Input: part model. Units: mm. Frame: model coordinates. Face numbers are marked on the shaded views. A direction names the side the tool comes from. Round coordinates to 2 decimals unless told otherwise and drop trailing zeros. Order: outer loops, then holes, each group sorted by start corner. A loop starts at its lowest first (then second) coordinate and runs counter-clockwise, first axis right, second up. Notation, with made-up numbers: M 0,73.5 L 23,73.5 A37 cw 23,110.5 Z; hole C 24,-22.75 d7. An arc over 180 degrees is marked long. One line per question, with ' | ' between items.
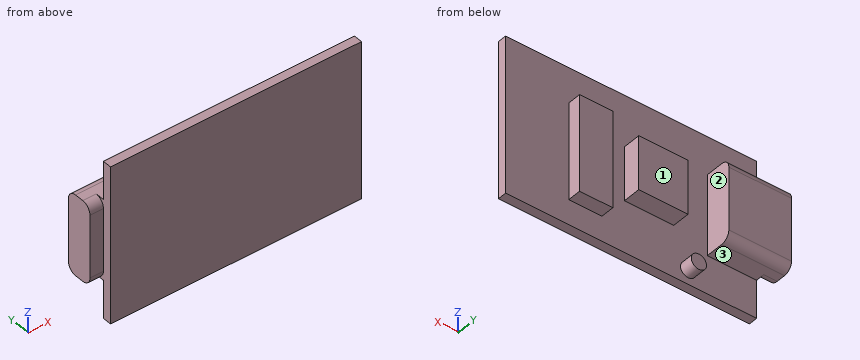
```python
from build123d import *

# Parameters (mm, degrees)
SKETCH1_W           = 28
SKETCH1_H           = 17.5
BOSS_EXTRUDE1_DEPTH = 1
SKETCH2_W           = 7
SKETCH2_H           = 9
BOSS_EXTRUDE2_DEPTH = 3
FILLET1_R           = 1
SKETCH3_W           = 5.5
SKETCH3_H           = 6
BOSS_EXTRUDE3_DEPTH = 2
SKETCH4_R           = 0.852579897
SKETCH4_W           = 3.701013581
SKETCH4_H           = 10.765249821
BOSS_EXTRUDE5_DEPTH = 1.5


with BuildPart() as part:
    # Sketch1 → Boss-Extrude1 (new body)
    with BuildSketch(Plane(origin=(0, 0, 0), x_dir=(1, 0, 0), z_dir=(0, 1, 0))):
        Rectangle(SKETCH1_W, SKETCH1_H)
    extrude(amount=BOSS_EXTRUDE1_DEPTH)

    # Sketch2 → Boss-Extrude2 (add)
    with BuildSketch(Plane(origin=(0, 1, 0), x_dir=(1, 0, 0), z_dir=(0, 1, 0))):
        with Locations((-12, 0)):
            Rectangle(SKETCH2_W, SKETCH2_H)
    extrude(amount=BOSS_EXTRUDE2_DEPTH)

    # Fillet1
    fillet1_edges = [part.edges().sort_by_distance(p)[0] for p in [
        (-14.75, 1, 4.5),
        (-14.75, 1, -4.5),
        (-12, 4, 4.5),
        (-12, 4, -4.5),
    ]]
    fillet(fillet1_edges, radius=FILLET1_R)

    # Sketch3 → Boss-Extrude3 (add)
    with BuildSketch(Plane(origin=(0, 1, 0), x_dir=(1, 0, 0), z_dir=(0, 1, 0))):
        with Locations((-2, 0)):
            Rectangle(SKETCH3_W, SKETCH3_H)
    extrude(amount=BOSS_EXTRUDE3_DEPTH)

    # Sketch4 → Boss-Extrude5 (add)
    with BuildSketch(Plane(origin=(0, 1, 0), x_dir=(1, 0, 0), z_dir=(0, 1, 0))):
        with Locations(Location((-6.360266619, 7.174385454, 0), (0, 0, 90))):
            Circle(SKETCH4_R)
        with Locations((5.095251608, 0.572775911)):
            Rectangle(SKETCH4_W, SKETCH4_H)
    extrude(amount=BOSS_EXTRUDE5_DEPTH)


solid = part.part
```
Item 1: Section query C-C, the plane z = -1.5. Return loops of the section in (x, y), plus the area to 3 significant figures.
Report:
outline: M -15.5,1 L -14,1 L -14,0 L 14,0 L 14,1 L 6.95,1 L 6.95,2.5 L 3.24,2.5 L 3.24,1 L 0.75,1 L 0.75,3 L -4.75,3 L -4.75,1 L -8.5,1 L -8.5,4 L -15.5,4 Z | area: 65.6 mm²
Item 2: Access query for the marked faces 1, 2 and 3. Directions: +Z, -Z, +X, -X, +Y, -Y. A direction counts if a zero-diameter tool reaches every point of the face in a straight line with its end or side. Return the directions, or none.
Report:
face 1: +Z, -Z, +X, +Y | face 2: +Z, -Z, +Y | face 3: -Z, -X, +Y
Item 3: Section query A-A, the plane y = 1.5. Return loops of the section in (x, z), plus the area to 3 significant figures.
Report:
outline: M -15.5,-4.37 L -14,-4.37 L -14,-4.5 L -8.5,-4.5 L -8.5,4.5 L -14,4.5 L -14,4.37 L -15.5,4.37 Z; C -6.36,-7.17 d1.71; M -4.75,-3 L 0.75,-3 L 0.75,3 L -4.75,3 Z; M 3.24,-5.96 L 6.95,-5.96 L 6.95,4.81 L 3.24,4.81 Z | area: 138 mm²
Item 4: First-contact query: pin 1 (1 mm diameter, centred on x = -11.5, y = 3.5, fed in from +Z); pin 2 (1.6 mm diameter, centred on y = 2.5, z = 1, fed in from +X); pin 3 (5 mm diameter, centred on x = 0, z = 1, fed in from +Y). Flat tips, straight axial feed; report the tip coordinate or a pass-through.
Report:
pin 1: z = 4.5 | pin 2: x = 6.95 | pin 3: y = 3
Item 5: Section query D-D, the plane y = 3.6. Return loops of the section in (x, z).
Report:
outline: M -15.5,-4.3 L -8.5,-4.3 L -8.5,4.3 L -15.5,4.3 Z
Item 6: Section query B-B, the plane x = 5.75. Return loops of the section in (y, z), plus the area to 3 significant figures.
Report:
outline: M 0,-8.75 L 1,-8.75 L 1,-5.96 L 2.5,-5.96 L 2.5,4.81 L 1,4.81 L 1,8.75 L 0,8.75 Z | area: 33.6 mm²
Item 7: Line query: line 1 along X through (y, z) = (2.4, -1); line 2 along X through (y, z) = (2.6, 2.25); line 3 along X through (y, z) = (1.05, 4). Output: solid intervals per line, ascending. Write a range as from..to.
Report:
line 1: -15.5..-8.5, -4.75..0.75, 3.24..6.95 | line 2: -15.5..-8.5, -4.75..0.75 | line 3: -14..-8.5, 3.24..6.95
